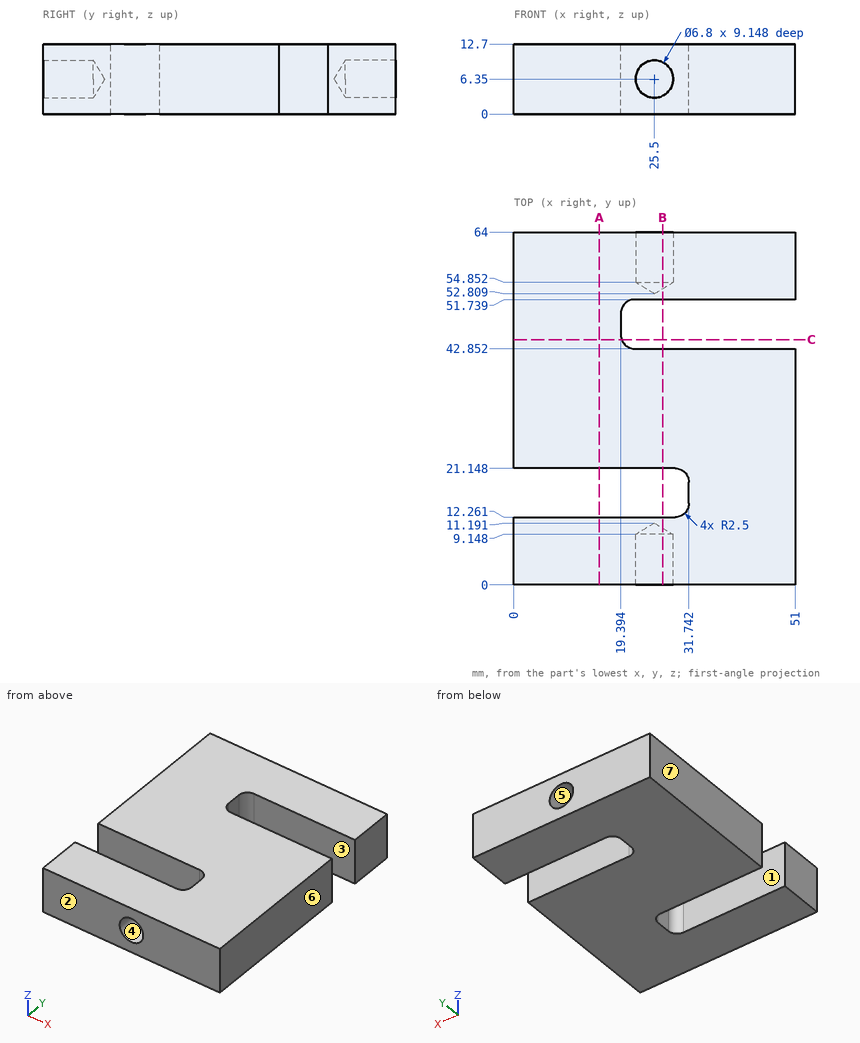
Geometry: see drawing. Coordinates: mm, zero at the bounding-box minimum. A direction names the side the tool comes from. Coordinates: 2 decimals unless noted, no trailing zeros. Loops run counter-clockwise (first coordinate to the right, second up) from the corner with the lowest first, then second, coordinate; pieces in that order, holes last. Notation, with made-up numbers: (-24.5, 22) -> (26.5, 22) arc R25 cw to (26.5, 51) -> close; hole circle Ø3 at (16.5, 28.25). An arc over 180 degrees is marked (long way). Write item = value, one per line. Start each with the question number.
Item 1: Cut plane B-B, the plane x = 27. Count the separate pieces of the cut face and the enclosed holes in it, plus the area to 3 significant figures.
Item 2: First-contact query: P1, Ø1.9, axis at y = 16.5, z = 6.5, coming from the -X side; P2, Ø3, axis at y = 46.5, z = 5.5, coming from the +X side; P3, Ø6, axis at x = 25.5, z = 6.35, coming from the -Y side. Flat tips, straight axial feed; report the tip coordinate or a pass-through.
Item 3: Material intervals for line 1 (Y direction, x = 24.5, z = 3); line 2 (Z direction, x = 25.5, y = 3.5); line 3 (Y direction, x = 24, z = 5.75), sorted ascending.
Item 4: Cut plane A-A, the plane x = 15.5. Return loops of the section in (y, z).
Item 5: Reachability of the marked faces 1, 2, 3 and 4 from +Z, -Z, +X, -X, +Y, -Y: full face, straight path, thin tool, end or side. Return the list, or none.
Item 6: Cut plane C-C, the plane y = 44.5. Return loops of the section in (x, z).
Item 7: Mould query, pull axis X, two halves, no side actions, for the marked faces 5, 6 and 7. Classes: pulls with the +X half, pulls with the -X half, needs draft (parallel to the pull), parting line crosses it, or undercut.
Ans:
q1.separate_pieces = 3
q1.enclosed_holes = 0
q1.area = 467 mm²
q2.P1 = 31.74
q2.P2 = 19.42
q2.P3 = 9.39
q3.line_1 = 0 to 12.26, 21.15 to 42.85, 51.74 to 64
q3.line_2 = 0 to 2.95, 9.75 to 12.7
q3.line_3 = 10.22 to 12.26, 21.15 to 42.85, 51.74 to 53.78
q4.outline = (0, 0) -> (12.26, 0) -> (12.26, 12.7) -> (0, 12.7) -> close; (21.15, 0) -> (64, 0) -> (64, 12.7) -> (21.15, 12.7) -> close
q5.face_1 = +Z, -Z, -X
q5.face_2 = +Z, -Z, +X, -X, -Y
q5.face_3 = +Z, -Z, +X
q5.face_4 = -Y
q6.outline = (0, 0) -> (19.54, 0) -> (19.54, 12.7) -> (0, 12.7) -> close
q7.face_5 = undercut
q7.face_6 = pulls with the +X half
q7.face_7 = pulls with the -X half
